Design review of the part built by this model. Coordinates are the model's own, in mm. Coordinates: 2 decimals unless noted, no trailing zeros. Write each loop counter-clockwise with the first axis right and the second up, starting at its lowest first coordinate (ties: lowest second). Pieces come first, ordered by that corner, then holes. Notation, with made-up numbers: (3, -19.5) - (55, -19.5) arc R17 ccw to (55, 7.5) - close; hole circle Ø2 at (87.25, 49). An arc over 180 degrees is marked (long way). One line per item, written item: value.
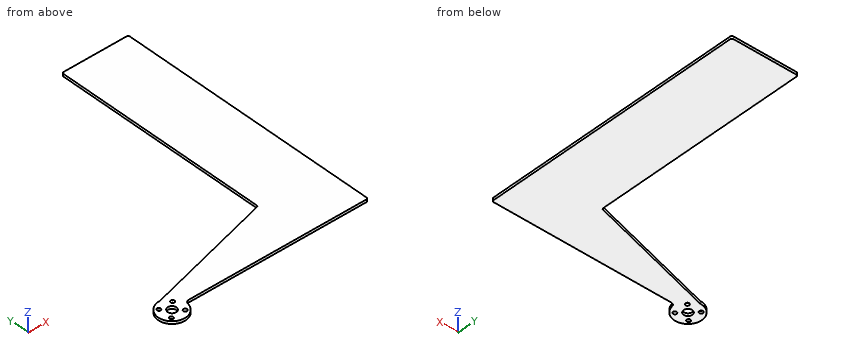
from build123d import *

# Parameters (mm, degrees)
SKETCH_R   = 2.15
SKETCH_R_2 = 5
PAD_DEPTH  = 3


with BuildPart() as part:
    # Sketch → Pad (new body)
    with BuildSketch(Plane.XY):
        with BuildLine():
            Line((36.7, 0.5), (225.5, 0.5))
            ThreePointArc((225.5, 0.5), (226.914214, 1.085786), (227.5, 2.5))
            Line((227.5, 2.5), (227.5, 303.3))
            ThreePointArc((227.5, 303.3), (226.914214, 304.714214), (225.5, 305.3))
            Line((225.5, 305.3), (152.7, 305.3))
            ThreePointArc((152.7, 305.3), (151.285786, 304.714214), (150.7, 303.3))
            Line((150.7, 303.3), (150.7, 57.773493))
            ThreePointArc((149.217638, 55.841641), (150.286707, 56.55597), (150.7, 57.773493))
            Line((1.035276, 16.136297), (149.217638, 55.841641))
            ThreePointArc((0, 16), (0.522105, 16.034221), (1.035276, 16.136297))
            ThreePointArc((0, 16), (-12.263768, -10.276186), (15.753095, -2.8))
            ThreePointArc((19.691369, 0.5), (17.122322, -0.434058), (15.753095, -2.8))
            Line((36.7, 0.5), (19.691369, 0.5))
        make_face()
        with Locations((-8, 8)):
            Circle(SKETCH_R, mode=Mode.SUBTRACT)
        with Locations((8, 8)):
            Circle(SKETCH_R, mode=Mode.SUBTRACT)
        with Locations((-8, -8)):
            Circle(SKETCH_R, mode=Mode.SUBTRACT)
        with Locations((8, -8)):
            Circle(SKETCH_R, mode=Mode.SUBTRACT)
        Circle(SKETCH_R_2, mode=Mode.SUBTRACT)
    extrude(amount=PAD_DEPTH)


solid = part.part
1. Insertion check: pin 1 Ø5 at (x, y) = (8, -8) entering from -Z; pin 2 Ø1.5 at (x, z) = (95, 1) entering from -Y. Each pin has a flat end and moves straight along its axis. Give the tip position at first contact, or say it passes through.
Answer block:
pin 1: stops at z = 0
pin 2: stops at y = 0.5
2. Consider section A-A, the plane z = 1.7. Write out the cut boundary in (x, y), then the cut area to 3 significant figures.
Answer block:
outline: (0, 16) arc R16 ccw (long way) to (15.75, -2.8) arc R4 cw to (19.69, 0.5) - (225.5, 0.5) arc R2 ccw to (227.5, 2.5) - (227.5, 303.3) arc R2 ccw to (225.5, 305.3) - (152.7, 305.3) arc R2 ccw to (150.7, 303.3) - (150.7, 57.77) arc R2 cw to (149.22, 55.84) - (1.04, 16.14) arc R4 cw to start; hole circle Ø4.3 at (-8, -8); hole circle Ø4.3 at (-8, 8); hole circle Ø10 at (0, 0); hole circle Ø4.3 at (8, -8); hole circle Ø4.3 at (8, 8)
area: 29,200 mm^2
3. Wall thickness on line 1 along Y through (x, z) = (0, 1.3); line 2 along Y through (x, z) = (8, 1.9); line 3 along Y through (x, z) = (-8, 1.4): over which ranges is each line inside the solid? List them lowest first.
Answer block:
line 1: y = -16 to -5, 5 to 16
line 2: y = -13.86 to -10.15, -5.85 to 5.85, 10.15 to 18
line 3: y = -13.86 to -10.15, -5.85 to 5.85, 10.15 to 13.86
4. Consider section C-C, the plane y = 116. Write out the cut boundary in (x, z).
Answer block:
outline: (150.7, 0) - (227.5, 0) - (227.5, 3) - (150.7, 3) - close
5. Consider section B-B, the plane x = 196. Write out the cut boundary in (y, z).
Answer block:
outline: (0.5, 0) - (305.3, 0) - (305.3, 3) - (0.5, 3) - close
